```python
from build123d import *

# Parameters (mm, degrees)
BOSS_EXTRUDE1_DEPTH      = 10
BOSS_EXTRUDE1_DEPTH_BACK = 10


with BuildPart() as part:
    # Sketch1 → Boss-Extrude1 (new, two sides: drawn at the far end of the back side and taken through both)
    with BuildSketch(Plane.XY.offset(-BOSS_EXTRUDE1_DEPTH_BACK)):
        Polygon((7.274522478, 125.455869207), (22.274260332, 125.544550227), (22.25061206, 129.544480321), (18.250681966, 129.520832049), (18.227033694, 133.520762144), (22.226963788, 133.544410415), (22.203315516, 137.54434051), (7.203577663, 137.45565949), (7.227225935, 133.455729396), (11.227156029, 133.479377668), (11.250804301, 129.479447574), (7.250874206, 129.455799302), align=None)
    extrude(amount=BOSS_EXTRUDE1_DEPTH + BOSS_EXTRUDE1_DEPTH_BACK)


solid = part.part
```
Can you work these out from the model? Positions are in its coordinate system, mm. Coordinates: 2 decimals unless noted, no trailing zeros. Order: outer loops, then holes, each group sorted by start corner. A loop starts at its lowest first (then second) coordinate and runs counter-clockwise, first axis right, second up. Notation, with made-up numbers: (67, -25) - (94, -25) arc R24 cw to (94, -12) - close; hole circle Ø7 at (-38, 37). An arc over 180 degrees is marked (long way). Answer in a Markdown table with one row per item.
1. Suppose I cut it at B-B (z = -6). Please give me the cut outline in (x, y), and give its area (3 significant figures).
Reply:
| item | result |
|---|---|
| outline | (7.2, 137.46) - (7.23, 133.46) - (11.23, 133.48) - (11.25, 129.48) - (7.25, 129.46) - (7.27, 125.46) - (22.27, 125.54) - (22.25, 129.54) - (18.25, 129.52) - (18.23, 133.52) - (22.23, 133.54) - (22.2, 137.54) - close |
| area | 148 mm^2 |
2. Suppose I cut it at A-A (x = 8.25). Please give me the cut outline in (y, z), and give its area (3 significant figures).
Reply:
| item | result |
|---|---|
| outline | (125.46, -10) - (129.46, -10) - (129.46, 10) - (125.46, 10) - close; (133.46, -10) - (137.46, -10) - (137.46, 10) - (133.46, 10) - close |
| area | 160 mm^2 |
3. For pin 1 (5 mm diameter, centred on y = 133, z = -6.5, fed in from +X); pin 2 (4 mm diameter, centred on y = 135, z = -4.5, fed in from -X); pin 3 (3 mm diameter, centred on y = 128.5, z = 0, fed in from -X), each with a flat end and sliding along its axis, tell me the tip position at first contact or that it passes through.
Reply:
| item | result |
|---|---|
| pin 1 | stops at x = 22.23 |
| pin 2 | stops at x = 7.21 |
| pin 3 | stops at x = 7.25 |
4. Suppose I cut it at C-C (y = 130.75). Please give me the cut outline in (x, z).
Reply:
| item | result |
|---|---|
| outline | (11.24, -10) - (18.24, -10) - (18.24, 10) - (11.24, 10) - close |
5. If I drill on line 1 along Y through (x, z) = (21.75, 5); line 2 along X through (y, z) = (132.5, -6); line 3 along X through (y, z) = (134, -5.25), over which ranges is the centre line in solid material (lowest first)?
Reply:
| item | result |
|---|---|
| line 1 | y = 125.54 to 129.54, 133.54 to 137.54 |
| line 2 | x = 11.23 to 18.23 |
| line 3 | x = 7.22 to 22.22 |
